Geometry check sheet. Reference: the model listing, model coordinates, mm. Give positions to 0.01 mm unless a question says otherwise; leave off trailing zeros.
1. Material ranges on L1, parallel to Y at x = 9, z = 4.75 (1 decimal); L2, parallel to X at y = 60, z = 6 (3 decimals); L3, parallel to Y at x = -49, z = 5.5 (3 decimals), recorded low to high.
2. Release check for a two-part mould opening along Y. For faces 1 (the flat face through (-2, 2, 6.35)), 2 (the flat face through (-2, 111.125, 3)), 3 (the cylindrical face through (-33.11, -55.583, 3.131)) record: +Y half, -Y half, draft (parallel to the pull), parting line (faces both ways), or undercut.
3. Go/stop test with a flat-tipped pin: pin 1 Ø4.5 at (x, y) = (10, 14.56) entering from -Z. Record where the tip stops, or that it passes through.
from build123d import *

# Parameters (mm, degrees)
F0_W     = 222.25
F0_H     = 222.25
F0_R     = 1.5875
F0_R_2   = 2.38125
F1_DEPTH = 6.35


with BuildPart() as f1:
    # F0 (on Top) → F1 (new body)
    with BuildSketch(Plane.XY):
        Rectangle(F0_W, F0_H)
        with Locations((-104.775, -104.775)):
            Circle(F0_R, mode=Mode.SUBTRACT)
        with Locations((-50.8, -81.94375)):
            Circle(F0_R_2, mode=Mode.SUBTRACT)
        with Locations((-32.8, -81.94375)):
            Circle(F0_R_2, mode=Mode.SUBTRACT)
        with Locations((-50.8, -57.94375)):
            Circle(F0_R_2, mode=Mode.SUBTRACT)
        with Locations((-32.8, -57.94375)):
            Circle(F0_R_2, mode=Mode.SUBTRACT)
        with Locations((32.8, -81.94375)):
            Circle(F0_R_2, mode=Mode.SUBTRACT)
        with Locations((50.8, -81.94375)):
            Circle(F0_R_2, mode=Mode.SUBTRACT)
        with Locations((32.8, -57.94375)):
            Circle(F0_R_2, mode=Mode.SUBTRACT)
        with Locations((50.8, -57.94375)):
            Circle(F0_R_2, mode=Mode.SUBTRACT)
        with Locations((104.775, -104.775)):
            Circle(F0_R, mode=Mode.SUBTRACT)
        with Locations((-10, 14.55625)):
            Circle(F0_R_2, mode=Mode.SUBTRACT)
        with Locations((-104.775, 104.775)):
            Circle(F0_R, mode=Mode.SUBTRACT)
        with Locations((-9, 57.94375)):
            Circle(F0_R_2, mode=Mode.SUBTRACT)
        with Locations((-9, 81.94375)):
            Circle(F0_R_2, mode=Mode.SUBTRACT)
        with Locations((10, 14.55625)):
            Circle(F0_R_2, mode=Mode.SUBTRACT)
        with Locations((9, 57.94375)):
            Circle(F0_R_2, mode=Mode.SUBTRACT)
        with Locations((9, 81.94375)):
            Circle(F0_R_2, mode=Mode.SUBTRACT)
        with Locations((104.775, 104.775)):
            Circle(F0_R, mode=Mode.SUBTRACT)
    extrude(amount=F1_DEPTH)


solid = f1.part
Result:
1. L1: y = -111.1 to 12.4, 16.7 to 55.6, 60.3 to 79.6, 84.3 to 111.1
1. L2: x = -111.125 to -10.201, -7.799 to 7.799, 10.201 to 111.125
1. L3: y = -111.125 to -83.503, -80.385 to -59.503, -56.385 to 111.125
2. face 1: draft
2. face 2: +Y half
2. face 3: undercut
3. pin 1: passes through
